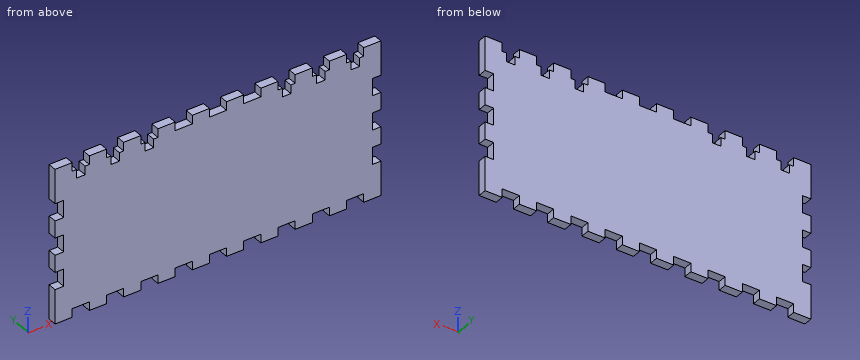
```python
from build123d import *

# Parameters (mm, degrees)
SKETCH1_W           = 241.3
SKETCH1_H           = 114.3
BOSS_EXTRUDE1_DEPTH = 6.35
SKETCH2_W           = 12.7
SKETCH2_H           = 6.35
CUT_EXTRUDE1_DEPTH  = 7.35
SKETCH3_W           = 6.35
SKETCH3_H           = 12.7
CUT_EXTRUDE2_DEPTH  = 7.35
LPATTERN1_COUNT     = 2
LPATTERN1_PITCH     = 25.4
LPATTERN1_COL_COUNT = 2
LPATTERN1_COL_PITCH = 25.4
SKETCH4_W           = 6.35
SKETCH4_H           = 6.35
CUT_EXTRUDE3_DEPTH  = 7.35
LPATTERN2_COUNT     = 9
LPATTERN2_PITCH     = 25.4


with BuildPart() as part:
    # Sketch1 → Boss-Extrude1 (new body)
    with BuildSketch(Plane(origin=(0, 0, 0), x_dir=(1, 0, 0), z_dir=(0, 1, 0))):
        with Locations((120.65, 57.15)):
            Rectangle(SKETCH1_W, SKETCH1_H)
    extrude(amount=BOSS_EXTRUDE1_DEPTH)

    # Sketch2 → Cut-Extrude1 (cut, through all)
    with BuildSketch(Plane(origin=(0, 6.35, 0), x_dir=(1, 0, 0), z_dir=(0, 1, 0))):
        with Locations((19.05, 111.125)):
            Rectangle(SKETCH2_W, SKETCH2_H)
        with Locations((-6.35, 111.125)):
            Rectangle(SKETCH2_W, SKETCH2_H)
        with Locations((-6.35, 3.175)):
            Rectangle(SKETCH2_W, SKETCH2_H)
        with Locations((19.05, 3.175)):
            Rectangle(SKETCH2_W, SKETCH2_H)
        with Locations((44.45, 111.125)):
            Rectangle(SKETCH2_W, SKETCH2_H)
        with Locations((44.45, 3.175)):
            Rectangle(SKETCH2_W, SKETCH2_H)
        with Locations((69.85, 111.125)):
            Rectangle(SKETCH2_W, SKETCH2_H)
        with Locations((69.85, 3.175)):
            Rectangle(SKETCH2_W, SKETCH2_H)
        with Locations((95.25, 111.125)):
            Rectangle(SKETCH2_W, SKETCH2_H)
        with Locations((95.25, 3.175)):
            Rectangle(SKETCH2_W, SKETCH2_H)
        with Locations((120.65, 111.125)):
            Rectangle(SKETCH2_W, SKETCH2_H)
        with Locations((120.65, 3.175)):
            Rectangle(SKETCH2_W, SKETCH2_H)
        with Locations((146.05, 111.125)):
            Rectangle(SKETCH2_W, SKETCH2_H)
        with Locations((146.05, 3.175)):
            Rectangle(SKETCH2_W, SKETCH2_H)
        with Locations((171.45, 111.125)):
            Rectangle(SKETCH2_W, SKETCH2_H)
        with Locations((171.45, 3.175)):
            Rectangle(SKETCH2_W, SKETCH2_H)
        with Locations((196.85, 111.125)):
            Rectangle(SKETCH2_W, SKETCH2_H)
        with Locations((196.85, 3.175)):
            Rectangle(SKETCH2_W, SKETCH2_H)
        with Locations((222.25, 111.125)):
            Rectangle(SKETCH2_W, SKETCH2_H)
        with Locations((222.25, 3.175)):
            Rectangle(SKETCH2_W, SKETCH2_H)
    extrude(amount=-CUT_EXTRUDE1_DEPTH, mode=Mode.SUBTRACT)

    # Sketch3 → Cut-Extrude2 (cut, through all)
    with BuildSketch(Plane(origin=(0, 6.35, 0), x_dir=(1, 0, 0), z_dir=(0, 1, 0))):
        with Locations((3.175, 57.15)):
            Rectangle(SKETCH3_W, SKETCH3_H)
        with Locations((238.125, 57.15)):
            Rectangle(SKETCH3_W, SKETCH3_H)
    cut_extrude2 = extrude(amount=-CUT_EXTRUDE2_DEPTH, mode=Mode.SUBTRACT)

    # LPattern1: Cut-Extrude2 ×2
    with Locations(*[(0, 0, i * LPATTERN1_PITCH) for i in range(1, LPATTERN1_COUNT)]):
        add(cut_extrude2, mode=Mode.SUBTRACT)

    # LPattern1 col: Cut-Extrude2 ×2
    with Locations(*[(0, 0, -i * LPATTERN1_COL_PITCH) for i in range(1, LPATTERN1_COL_COUNT)]):
        add(cut_extrude2, mode=Mode.SUBTRACT)

    # Sketch4 → Cut-Extrude3 (cut, through all)
    with BuildSketch(Plane(origin=(0, 6.35, 0), x_dir=(1, 0, 0), z_dir=(0, 1, 0))):
        with Locations((19.05, 9.525)):
            Rectangle(SKETCH4_W, SKETCH4_H)
    cut_extrude3 = extrude(amount=-CUT_EXTRUDE3_DEPTH, mode=Mode.SUBTRACT)

    # LPattern2: Cut-Extrude3 ×9, 3 skipped
    with Locations(*[(i * LPATTERN2_PITCH, 0, 0) for i in range(1, LPATTERN2_COUNT) if i not in (3, 4, 5)]):
        add(cut_extrude3, mode=Mode.SUBTRACT)


solid = part.part
```
Read the model definition and answer for the solid it produces. Units are mm, in the model's axes. Give positions to 0.01 mm unless a question says otherwise; leave off trailing zeros. Write each loop counter-clockwise with the first axis right and the second up, starting at its lowest first coordinate (ties: lowest second). Pieces come first, ordered by that corner, then holes. Notation, with made-up numbers: (65.25, 38.25) - (77.25, 38.25) arc R5 cw to (77.25, 42.25) - close; hole circle Ø4 at (16, -35.5). An arc over 180 degrees is marked (long way). Write item = value, one per line. Start each with the question number.
Item 1: Find section B-B (x = 19.5). Give the vertices of the cut face in (y, z).
Item 2: Find section A-A (z = -34.5). Give the vertices of the cut face in (x, y).
Item 3: Find the intervals of material crossed by probe 1 along Z at (x, y) = (17, 3.75); probe 2 along X at (y, z) = (2, -59); probe 3 along Z at (x, y) = (93, 2.75), in increasing order. Write a range as [from, to].
Item 4: Each of these flat-tipped pins is pushed along its axis until it touches: P1, Ø1.9, axis at x = 143.5, y = 4.5, coming from the +Z side; P2, Ø1.9, axis at y = 3.5, z = -59.5, coming from the +X side; P3, Ø1.9, axis at x = 171, y = 4.5, coming from the +Z side. Where does it stop, or does it pass through?
Response:
q1.outline = (0, -107.95) - (6.35, -107.95) - (6.35, -12.7) - (0, -12.7) - close
q2.outline = (6.35, 0) - (234.95, 0) - (234.95, 6.35) - (6.35, 6.35) - close
q3.probe_1 = [-107.95, -12.7]
q3.probe_2 = [6.35, 234.95]
q3.probe_3 = [-107.95, -6.35]
q4.P1 = -6.35
q4.P2 = 234.95
q4.P3 = -12.7
